from build123d import *

# Parameters (mm, degrees)
BOSS_EXTRUDE1_DEPTH                             = 5
SKETCH5_W                                       = 1.78
SKETCH5_H                                       = 50
BOSS_EXTRUDE3_DEPTH                             = 1.5
BOSS_EXTRUDE4_REACH                             = 55.614
SKETCH5_3_W                                     = 1.78
SKETCH5_3_H                                     = 50
BOSS_EXTRUDE5_DEPTH                             = 1.5
FILLET1_R                                       = 2
CSK_FOR_M2_FLAT_HEAD_MACHINE_SCREW2_D           = 2.4
CSK_FOR_M2_FLAT_HEAD_MACHINE_SCREW2_CSINK_D     = 4.4
CSK_FOR_M2_FLAT_HEAD_MACHINE_SCREW2_CSINK_ANGLE = 90
CHAMFER1_SIZE                                   = 2
BOSS_EXTRUDE6_DEPTH                             = 1.5
LPATTERN1_COUNT                                 = 4
LPATTERN1_PITCH                                 = 16.166666667


with BuildPart() as part:
    # Sketch1 → Boss-Extrude1 (new body)
    with BuildSketch(Plane(origin=(0, 4, 0), x_dir=(1, 0, 0), z_dir=(0, 1, 0))):
        Polygon((-14.18, 46.928571429), (-14.18, 50), (-17.13, 50), (-17.13, 0), (-14.18, 0), (-14.18, 3.071428571), (-9.703639402, 3.071428571), (-5.570306069, 13.785714286), (-1.78, 13.785714286), (-1.78, 0), (0, 0), (0, 50), (-1.78, 50), (-1.78, 36.214285714), (-5.570306069, 36.214285714), (-9.703639402, 46.928571429), align=None)
        Polygon((-14.18, 4.071428571), (-14.18, 24.5), (-10.389693931, 24.5), (-6.449249487, 14.285714286), (-10.389693931, 4.071428571), align=None, mode=Mode.SUBTRACT)
        Polygon((-10.389693931, 45.928571429), (-6.449249487, 35.714285714), (-10.389693931, 25.5), (-14.18, 25.5), (-14.18, 45.928571429), align=None, mode=Mode.SUBTRACT)
        Polygon((-5.570306069, 14.785714286), (-9.510750513, 25), (-5.570306069, 35.214285714), (-1.78, 35.214285714), (-1.78, 14.785714286), align=None, mode=Mode.SUBTRACT)
    extrude(amount=BOSS_EXTRUDE1_DEPTH)

    # Sketch5_3 → Boss-Extrude4 (add, up to next)
    with BuildSketch(Plane.XZ, mode=Mode.PRIVATE) as boss_extrude4_sk1:
        with Locations((-0.89, -25)):
            Rectangle(SKETCH5_3_W, SKETCH5_3_H)
    boss_extrude4_tool1 = extrude(boss_extrude4_sk1.sketch, amount=-BOSS_EXTRUDE4_REACH, mode=Mode.PRIVATE) - part.part


with BuildPart() as body_2:
    # Sketch5 → Boss-Extrude3 (new body)
    with BuildSketch(Plane.XZ):
        Polygon((12, -10), (7, -10), (7, -40), (12, -40), (12, -50), (0, -50), (0, 0), (12, 0), align=None)
        with Locations((-0.89, -25)):
            Rectangle(SKETCH5_W, SKETCH5_H)
    extrude(amount=BOSS_EXTRUDE3_DEPTH)


with BuildPart() as part_1:
    add(part.part)

    add(body_2.part)  # Boss-Extrude4 merges body 2
    add(boss_extrude4_tool1.solids().sort_by_distance((-0.89, 0, -25))[0])

    # Sketch7 → Boss-Extrude5 (add)
    with BuildSketch(Plane(origin=(0, 3.25, 0), x_dir=(1, 0, 0), z_dir=(0, 1, 0))):
        Polygon((12, 40), (12, 50), (0, 50), (0, 0), (12, 0), (12, 10), (7, 10), (7, 40), align=None)
    extrude(amount=BOSS_EXTRUDE5_DEPTH)

    # Fillet1
    fillet1_edges = [part_1.edges().sort_by_distance(p)[0] for p in [
        (7, -0.75, -10),
        (12, -0.75, -10),
        (12, -0.75, 0),
        (12, -0.75, -50),
        (12, -0.75, -40),
        (7, -0.75, -40),
        (12, 4, -50),
        (12, 4, 0),
        (12, 4, -10),
        (7, 4, -10),
        (7, 4, -40),
        (12, 4, -40),
    ]]
    fillet(fillet1_edges, radius=FILLET1_R)

    # CSK for M2 Flat Head Machine Screw2 (through all)
    with Locations(Plane(origin=(0, -1.5, 0), x_dir=(-1, 0, 0), z_dir=(0, -1, 0))):
        with Locations((-7, 45), (-7, 5)):
            CounterSinkHole(CSK_FOR_M2_FLAT_HEAD_MACHINE_SCREW2_D / 2, CSK_FOR_M2_FLAT_HEAD_MACHINE_SCREW2_CSINK_D / 2, counter_sink_angle=CSK_FOR_M2_FLAT_HEAD_MACHINE_SCREW2_CSINK_ANGLE)

    # Chamfer1
    chamfer1_edges = [part_1.edges().sort_by_distance(p)[0] for p in [
        (-17.13, 9, -25),
    ]]
    chamfer(chamfer1_edges, length=CHAMFER1_SIZE)

    # Sketch11 → Boss-Extrude6 (add)
    with BuildSketch(Plane.XY):
        Polygon((0, 9), (0, 4.75), (4.25, 4.75), align=None)
    boss_extrude6 = extrude(amount=-BOSS_EXTRUDE6_DEPTH)

    # LPattern1: Boss-Extrude6 ×4
    with Locations(*[(0, 0, -i * LPATTERN1_PITCH) for i in range(1, LPATTERN1_COUNT)]):
        add(boss_extrude6)


solid = part_1.part
Geometry: final body of the model. Coordinates: model frame, mm. A direction names the side the tool comes from. Give positions to 0.01 mm unless a question says otherwise; leave off trailing zeros. Write each loop counter-clockwise with the first axis right and the second up, starting at its lowest first coordinate (ties: lowest second). Pieces come first, ordered by that corner, then holes.
(1) Access query for faces 1 (the flat face through (-12, 6, -46.929)), 2 (the flat face through (1, 6, -48.5)), 3 (the flat face through (-12, 6, -25.5)), 4 (the flat face through (5, 0, -25)), 5 (the cylindrical face through (11.43, -0.76, -9.4)). Directions: +Z, -Z, +X, -X, +Y, -Y. A direction counts if a zero-diameter tool reaches every point of the face in a straight line with its end or side. Return the directions, or none.
(2) Cut plane A-A, the plane x = 2.5. Return loops of the section in (y, z), then the cut area to 4 significant figures.
(3) Mould query, pull axis Z, two halves, no side actions, for faces 6 (the flat face through (-4, 6, -13.786)), 7 (the flat face through (2, 7, -17)), 8 (the flat face through (-8.39, 6.46, -9.25)), 9 (the flat face through (-8.39, 6.46, -30.68)). Classes: released by +Z, released by -Z, zero draft, split by the parting line, or undercut.
(4) Cut plane C-C, the plane z = -29.5. Return loops of the section in (x, y).
(5) First-contact query: P1, Ø4.5, axis at x = 3, y = 6, coming from the +Z side; P2, Ø4, axis at x = 7, z = -5, coming from the +Y side; P3, Ø5, axis at x = -11.5, y = 5.5, coming from the -Z side; P4, Ø1.5, axis at x = -3, z = -11, coming from the -Y side. Flat tips, straight axial feed; report the tip coordinate or a pass-through.
(6) Cut plane D-D, the plane z = -5. Give the number of separate pieces and of enclosed holes in the cut face, then the cut area to 3 significant figures.
(7) Ray query, line 1 (Z direction, x = -13.25, y = 8.5); line 2 (Y direction, x = 5.75, z = -11); line 3 (X direction, y = -0.15, z = -45). Return the intervals inside material, ascending.
(8) Cut plane B-B, the plane x = -13.5. Return loops of the section in (y, z), then the cut area to 3 significant figures.
Values follow:
1. face 1: -Z, +Y, -Y
1. face 2: +X, +Y
1. face 3: +Y, -Y
1. face 4: +Z, -Z, +X
1. face 5: +X, +Y, -Y
2. outline: (-1.5, -50) - (0, -50) - (0, 0) - (-1.5, 0) - close; (3.25, -50) - (6.5, -50) - (6.5, -48.5) - (4.75, -48.5) - (4.75, -33.83) - (6.5, -33.83) - (6.5, -32.33) - (4.75, -32.33) - (4.75, -17.67) - (6.5, -17.67) - (6.5, -16.17) - (4.75, -16.17) - (4.75, -1.5) - (6.5, -1.5) - (6.5, 0) - (3.25, 0) - close
2. area: 160.5 mm2
3. face 6: released by +Z
3. face 7: zero draft
3. face 8: undercut
3. face 9: undercut
4. outline: (-17.13, 4) - (-14.18, 4) - (-14.18, 9) - (-15.13, 9) - (-17.13, 7) - close; (-8.85, 4) - (-7.77, 4) - (-7.77, 9) - (-8.85, 9) - close; (-1.78, -1.5) - (7, -1.5) - (7, 0) - (0, 0) - (0, 3.25) - (7, 3.25) - (7, 4.75) - (0, 4.75) - (0, 9) - (-1.78, 9) - close
5. P1: stops at z = 0
5. P2: stops at y = 4.75
5. P3: stops at z = -46.93
5. P4: passes through
6. separate pieces: 5
6. enclosed holes: 0
6. area: 64.6 mm2
7. line 1: z = -46.93 to -45.93, -25.5 to -24.5, -4.07 to -3.07
7. line 2: y = -1.5 to 0, 3.25 to 4.75
7. line 3: x = -1.78 to 5.8, 8.2 to 12
8. outline: (4, -46.93) - (9, -46.93) - (9, -45.93) - (4, -45.93) - close; (4, -25.5) - (9, -25.5) - (9, -24.5) - (4, -24.5) - close; (4, -4.07) - (9, -4.07) - (9, -3.07) - (4, -3.07) - close
8. area: 15.0 mm2
